from build123d import *
from OCP.BRepFilletAPI import BRepFilletAPI_MakeChamfer

# Parameters (mm, degrees)
BOSS_EXTRUDE1_DEPTH      = 10
BOSS_EXTRUDE1_DEPTH_BACK = 24.004
SKETCH1_R                = 2.5
CUT_EXTRUDE1_START       = -80
SKETCH2_R                = 3.5
SKETCH2_R_2              = 1.75
SKETCH2_R_3              = 1.25
CUT_EXTRUDE1_DEPTH       = 26.835684039
CUT_EXTRUDE2_START       = -75.5
SKETCH2_6_R              = 1.75
SKETCH2_6_R_2            = 1.25
CUT_EXTRUDE2_DEPTH       = 31.33568418
CUT_EXTRUDE3_START       = -74.5
SKETCH2_7_R              = 1.25
CUT_EXTRUDE3_DEPTH       = 15
SKETCH3_W                = 57.958934366
SKETCH3_H                = 38.963082507
CUT_EXTRUDE4_DEPTH       = 106.83568418
CUT_EXTRUDE5_START       = -25
SKETCH4_R                = 3.175
CUT_EXTRUDE5_DEPTH       = 22.5
SKETCH4_2_R              = 3.175
CUT_EXTRUDE6_DEPTH       = 115.351178616
CHAMFER1_SIZE            = 0.5
CHAMFER1_SIZE2           = 1.366025404


with BuildPart() as part:
    # Sketch1 → Boss-Extrude1 (new, two sides: drawn at the far end of the back side and taken through both)
    with BuildSketch(Plane(origin=(0, 0, 0), x_dir=(1, 0, 0), z_dir=(0, 1, 0)).offset(-BOSS_EXTRUDE1_DEPTH_BACK)):
        with BuildLine():
            Line((-25, 74.5), (-25, -74.5))
            Line((-25, -74.5), (-6.330284354, -74.5))
            ThreePointArc((-6.330284354, -74.5), (0, -68.65), (6.330284354, -74.5))
            ThreePointArc((6.330284354, -74.5), (6.345069174, -74.749805722), (6.35, -75))
            ThreePointArc((6.35, -75), (6.345069174, -75.250194278), (6.330284354, -75.5))
            ThreePointArc((6.330284354, -75.5), (0, -81.35), (-6.330284354, -75.5))
            Line((-6.330284354, -75.5), (-24.9949995, -75.5))
            ThreePointArc((-24.9949995, -75.5), (0, -100), (24.9949995, -75.5))
            ThreePointArc((24.9949995, -75.5), (24.998749844, -75.250012502), (25, -75))
            Line((25, -75), (25, 75))
            ThreePointArc((25, 75), (24.998749844, 75.250012502), (24.9949995, 75.5))
            ThreePointArc((24.9949995, 75.5), (0, 100), (-24.9949995, 75.5))
            Line((-24.9949995, 75.5), (-6.330284354, 75.5))
            ThreePointArc((-6.330284354, 75.5), (0, 81.35), (6.330284354, 75.5))
            ThreePointArc((6.330284354, 75.5), (6.345069174, 75.250194278), (6.35, 75))
            ThreePointArc((6.35, 75), (6.345069174, 74.749805722), (6.330284354, 74.5))
            ThreePointArc((6.330284354, 74.5), (0, 68.65), (-6.330284354, 74.5))
            Line((-6.330284354, 74.5), (-25, 74.5))
        make_face()
        with Locations(Location((-15, -50, 0), (0, 0, 270))):
            Circle(SKETCH1_R, mode=Mode.SUBTRACT)
        with Locations(Location((15, -50, 0), (0, 0, 270))):
            Circle(SKETCH1_R, mode=Mode.SUBTRACT)
        with Locations(Location((-15, 50, 0), (0, 0, 270))):
            Circle(SKETCH1_R, mode=Mode.SUBTRACT)
        with Locations(Location((15, 50, 0), (0, 0, 270))):
            Circle(SKETCH1_R, mode=Mode.SUBTRACT)
    extrude(amount=BOSS_EXTRUDE1_DEPTH + BOSS_EXTRUDE1_DEPTH_BACK)

    # Sketch2 → Cut-Extrude1 (cut, through all)
    # profile 1 of 3: a face of its own
    with BuildSketch(Plane.XY.offset(CUT_EXTRUDE1_START)):
        with Locations((-15.67249975, 5)):
            Circle(SKETCH2_R)
        with Locations((-15.67249975, 5)):
            Circle(SKETCH2_R_2, mode=Mode.SUBTRACT)
    # profile 2 of 3: a face of its own
    with BuildSketch(Plane.XY.offset(CUT_EXTRUDE1_START)):
        with Locations((-15.67249975, 5)):
            Circle(SKETCH2_R_2)
        with Locations((-15.67249975, 5)):
            Circle(SKETCH2_R_3, mode=Mode.SUBTRACT)
    # profile 3 of 3: a face of its own
    with BuildSketch(Plane.XY.offset(CUT_EXTRUDE1_START)):
        with Locations((-15.67249975, 5)):
            Circle(SKETCH2_R_3)
    extrude(amount=-CUT_EXTRUDE1_DEPTH, mode=Mode.SUBTRACT)

    # Sketch2<6> → Cut-Extrude2 (cut, through all)
    # profile 1 of 2: a face of its own
    with BuildSketch(Plane.XY.offset(CUT_EXTRUDE2_START)):
        with Locations((-15.67249975, 5)):
            Circle(SKETCH2_6_R)
        with Locations((-15.67249975, 5)):
            Circle(SKETCH2_6_R_2, mode=Mode.SUBTRACT)
    # profile 2 of 2: a face of its own
    with BuildSketch(Plane.XY.offset(CUT_EXTRUDE2_START)):
        with Locations((-15.67249975, 5)):
            Circle(SKETCH2_6_R_2)
    extrude(amount=-CUT_EXTRUDE2_DEPTH, mode=Mode.SUBTRACT)

    # Sketch2<7> → Cut-Extrude3 (cut)
    with BuildSketch(Plane.XY.offset(CUT_EXTRUDE3_START)):
        with Locations((-15.67249975, 5)):
            Circle(SKETCH2_7_R)
    extrude(amount=CUT_EXTRUDE3_DEPTH, mode=Mode.SUBTRACT)

    # Sketch3 → Cut-Extrude4 (cut, through all)
    with BuildSketch(Plane.XY):
        with Locations((1.618964647, -7.082948233)):
            Rectangle(SKETCH3_W, SKETCH3_H)
    extrude(amount=CUT_EXTRUDE4_DEPTH, mode=Mode.SUBTRACT)

    # Mirror1: part across plane


with BuildPart() as part_1:
    add(part.part)
    add(part.part.mirror(Plane.XY))

    # Sketch4 → Cut-Extrude5 (cut)
    with BuildSketch(Plane.ZY.offset(25).offset(CUT_EXTRUDE5_START)):
        with BuildLine():
            Line((-25.980762114, 10), (25.980762114, 10))
            Line((25.980762114, 10), (12.990381057, -12.5))
            ThreePointArc((12.990381057, -12.5), (0, -20), (-12.990381057, -12.5))
            Line((-12.990381057, -12.5), (-25.980762114, 10))
        make_face()
        with Locations((0, -5)):
            Circle(SKETCH4_R, mode=Mode.SUBTRACT)
    extrude(amount=-CUT_EXTRUDE5_DEPTH, mode=Mode.SUBTRACT)

    # Sketch4<2> → Cut-Extrude6 (cut, through all)
    with BuildSketch(Plane.ZY.offset(25)):
        with Locations((0, -5)):
            Circle(SKETCH4_2_R)
    extrude(amount=-CUT_EXTRUDE6_DEPTH, mode=Mode.SUBTRACT)

    # Chamfer1: one chamfer whose edges measure the first distance from different faces: ONE call of the kernel's chamfer builder (chamfer() names one face for all edges)
    chamfer1_edges_1 = [part_1.edges().sort_by_distance(p)[0] for p in [
        (15, -24.004, -52.5),
        (0.250012502, -24.004, 99.998749844),
        (-15.662641927, -24.004, 75.5),
        (-15, 10, 52.5),
        (15, 10, 52.5),
        (-15.665142177, 10, 74.5),
        (0.5, 10, 81.330284354),
        (-15.665142177, -24.004, 74.5),
        (0.5, -24.004, 81.330284354),
        (-17.42249975, 5, 75.5),
        (-15.662641927, 10, 75.5),
        (-15, -24.004, 52.5),
        (15, -24.004, 52.5),
        (0.250012502, 10, 99.998749844),
        (-17.42249975, 5, 80),
        (-16.92249975, 5, 74.5),
        (0, -5, -3.175),
        (25, -7.24506403, 2.24506403),
        (-25, -2.75493597, 2.24506403),
        (-15, -24.004, -52.5),
        (0.250012502, -24.004, -99.998749844),
        (0.5, 10, -81.330284354),
        (-15.665142177, 10, -74.5),
        (-15.662641927, -24.004, -75.5),
        (-15, 10, -52.5),
        (15, 10, -52.5),
        (0.250012502, 10, -99.998749844),
        (-15.662641927, 10, -75.5),
        (0.5, -24.004, -81.330284354),
        (-15.665142177, -24.004, -74.5),
        (-17.42249975, 5, -80),
        (-17.42249975, 5, -75.5),
        (-16.92249975, 5, -74.5),
        (-16.92249975, 5, -59.5),
        (25, 10, -37.5),
        (-25, 10, -37.25),
        (25, -24.004, 37.5),
        (-25, -24.004, -37.25),
    ]]
    chamfer1_edges_2 = [part_1.edges().sort_by_distance(p)[0] for p in [
        (11.25, 10, -25.980762114),
    ]]
    chamfer1_side_2 = [part_1.faces().sort_by_distance(p)[0] for p in [
        (-1.58584153, 10, 0),
    ]]
    chamfer1_edges_3 = [part_1.edges().sort_by_distance(p)[0] for p in [
        (11.25, 10, 25.980762114),
    ]]
    chamfer1_side_3 = [part_1.faces().sort_by_distance(p)[0] for p in [
        (11.25, -1.25, 19.485571585),
    ]]
    chamfer1 = BRepFilletAPI_MakeChamfer(part_1.part.solid().wrapped)
    for e in chamfer1_edges_1:
        chamfer1.Add(CHAMFER1_SIZE, e.wrapped)
    for e in chamfer1_edges_2:
        chamfer1.Add(CHAMFER1_SIZE, CHAMFER1_SIZE2, e.wrapped, chamfer1_side_2[0].wrapped)  # the first distance lies on this face
    for e in chamfer1_edges_3:
        chamfer1.Add(CHAMFER1_SIZE, CHAMFER1_SIZE2, e.wrapped, chamfer1_side_3[0].wrapped)  # the first distance lies on this face
    add(Compound.cast(chamfer1.Shape()), mode=Mode.REPLACE)


solid = part_1.part
The listing builds one solid part. Answer for the finished solid, in the listing's coordinates (mm). A direction names the side the tool comes from. Round coordinates to 2 decimals unless told otherwise and drop trailing zeros. Order: outer loops, then holes, each group sorted by start corner. A loop starts at its lowest first (then second) coordinate and runs counter-clockwise, first axis right, second up. Notation, with made-up numbers: (37.25, 22) - (79.25, 22) arc R23 ccw to (79.25, 35) - close; hole circle Ø2 at (87, 75). An arc over 180 degrees is marked (long way). Write item = value, one per line. Start each with the question number.
1) For a pull along Y with two mould halves and no side action, classify faces 1 (the flat face through (0, -24.004, 1)), 2 (the flat face through (-13, 5, 80)), 3 (the flat face through (-16, -7, 74.5)) as released by +Y, released by -Y, zero draft, split by the parting line, or undercut.
2) Section B-B, the plane y = -5 is taken. Count the separate pieces of the cut face and the enclosed holes in it, plus the area to 3 significant figures.
3) Straight lines are drawn through the part: L1, parallel to X at y = -15, z = -50; L2, parallel to X at y = 2, z = -3.5; L3, parallel to Z at x = 5.5, y = -4.5. For each, find the intervals that lie inside material, in ascending order.
4) Section C-C, the plane z = 0 is taken. Write down the section's boundary in (x, y) (3 decimals).
5) Given pin 1 (2 mm diameter, centred on x = -15.67, y = 5, fed in from +Z); pin 2 (9.5 mm diameter, centred on x = -19, y = -14, fed in from +Z); pin 3 (1 mm diameter, centred on x = -19.5, y = -12.5, fed in from -Z); pin 4 (10 mm diameter, centred on y = -5, z = 0, fed in from -X), each flat-ended and moving along its own axis, determine where each tip first touches the part or whether it passes through.
6) For faces 4 (the flat face through (22.5, -1, 1)), 5 (the cylindrical face through (-17.061, 3.935, 77.726)), 6 (the flat face through (-13, 5, -80)), 7 (the flat face through (-16, -7, -74.5)), determine the directions among +Z, -Z, +X, -X, +Y, -Y from which every point of the face is accessible in a straight line to the end or side of a thin tool.
7) Section A-A, the plane z = 50 is taken. Write down the section's boundary in (x, y).
Results list:
q1.face_1 = released by -Y
q1.face_2 = undercut
q1.face_3 = zero draft
q2.separate_pieces = 2
q2.enclosed_holes = 4
q2.area = 8,140 mm^2
q3.L1 = -25 to -17.5, -12.5 to 12.5, 17.5 to 25
q3.L2 = -25 to 0, 22.5 to 25
q3.L3 = -99.39 to -78.17, -71.83 to -17.61, 17.61 to 71.83, 78.17 to 99.39
q4.outline = (-25, -23.504) - (-24.5, -24.004) - (24.5, -24.004) - (25, -23.504) - (25, -8.675) - (24.5, -8.175) - (22.5, -8.175) - (22.5, -20) - (0, -20) - (0, -8.675) - (-0.5, -8.175) - (-24.5, -8.175) - (-25, -8.675) - close; (-25, -1.325) - (-24.5, -1.825) - (-0.5, -1.825) - (0, -1.325) - (0, 10) - (-24.5, 10) - (-25, 9.5) - close; (22.5, -1.825) - (24.5, -1.825) - (25, -1.325) - (25, 9.5) - (24.5, 10) - (22.5, 10) - close
q5.pin_1 = 59.5
q5.pin_2 = 95.54
q5.pin_3 = -91.25
q5.pin_4 = -25
q6.face_4 = +Y
q6.face_5 = +Z
q6.face_6 = -Z
q6.face_7 = -X, +Y, -Y
q7.outline = (-25, -23.5) - (-24.5, -24) - (-18, -24) - (-17.5, -23.5) - (-17.5, 9.5) - (-18, 10) - (-24.5, 10) - (-25, 9.5) - close; (-12.5, -23.5) - (-12, -24) - (12, -24) - (12.5, -23.5) - (12.5, 9.5) - (12, 10) - (-12, 10) - (-12.5, 9.5) - close; (17.5, -23.5) - (18, -24) - (24.5, -24) - (25, -23.5) - (25, 9.5) - (24.5, 10) - (18, 10) - (17.5, 9.5) - close
